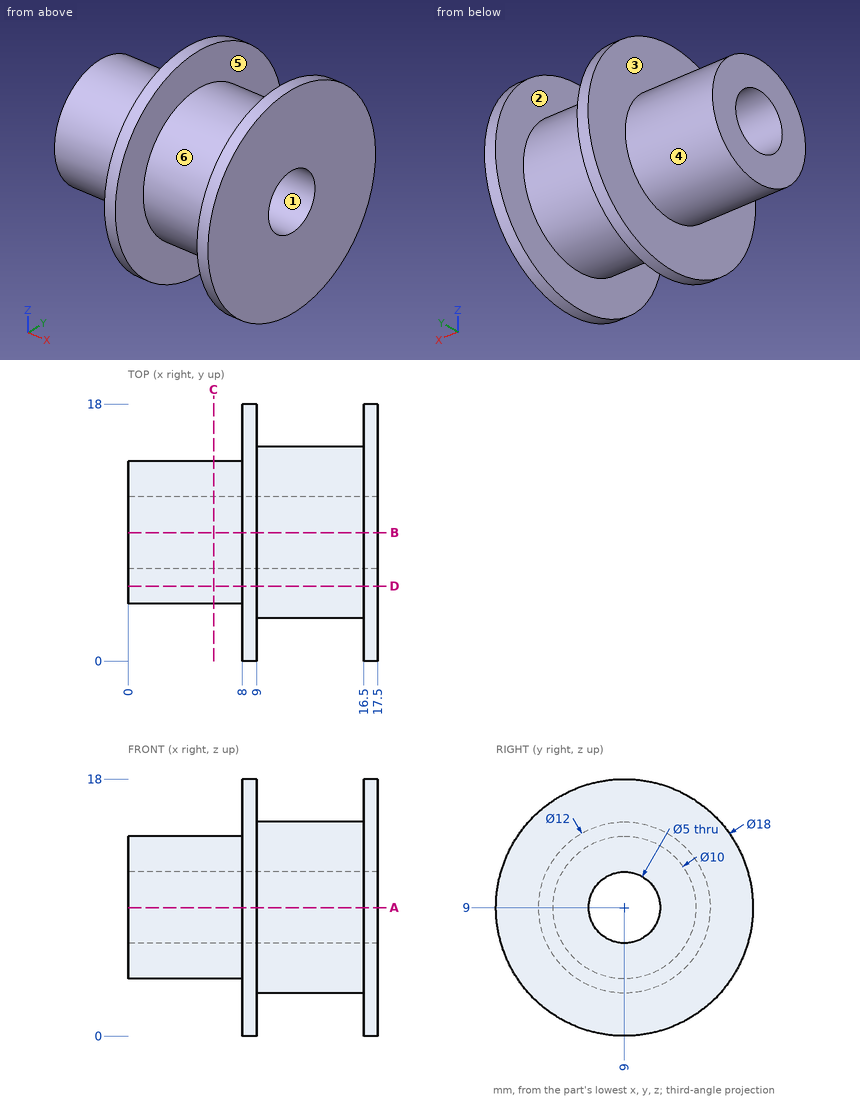
For this review, use the dimensioned drawing (mm, ordinates from the lowest corner) and the shaded views. A direction names the side the tool comes from. Round coordinates to 2 decimals unless told otherwise and drop trailing zeros. Order: outer loops, then holes, each group sorted by start corner. A loop starts at its lowest first (then second) coordinate and runs counter-clockwise, first axis right, second up. Notation, with made-up numbers: (10.25, -23) -> (53.25, -23) arc R15 cw to (53.25, -11) -> close; hole circle Ø3 at (-15.75, 52.5). An arc over 180 degrees is marked (long way). Write item = value, one per line. Start each with the question number.
Item 1: Consider section A-A on z = 9. Write out the cut boundary in (x, y), plus the area to 4 significant figures.
Item 2: Consider section C-C on x = 6. Write out the cut boundary in (y, z), plus the area to 3 significant figures.
Item 3: For the marked faces 1 and 2, list the 3-axis set-ups (+Z, -Z, +X, -X, +Y, -Y) from which the entire face can be reached by the end or side of a thin tool; tool diameter is ignored.
Item 4: Mouldability with a two-part tool opening along X and no side actions: class the marked faces 3, 4, 5 and 6 as released by +X, released by -X, zero draft, split by the parting line, or undercut.
Item 5: Consider section D-D on y = 5.25. Write out the cut boundary in (x, z), plus the area to 3 significant figures.
Item 6: Clearance check with flat-ended pins moving along their axes: pin 1 Ø3 at (x, z) = (5.5, 11.5) entering from +Y; pin 2 Ø5.5 at (y, z) = (7.5, 7.5) entering from -X; pin 3 Ø5 at (x, y) = (3.5, 4.5) entering from -Z; pin 4 Ø4 at (x, y) = (15.5, 2.5) entering from -Z. State where each tip first meets the part, or that it passes through.
Item 7: For line 1 along X through (y, z) = (15, 13.25); line 2 along X through (y, z) = (12.5, 4.5); line 3 along Z through (x, y) = (7.5, 8.25), list the stretches that pass through material, from the lowest coordinate up.
Conclusion:
q1.outline = (0, 4) -> (8, 4) -> (8, 0) -> (9, 0) -> (9, 3) -> (16.5, 3) -> (16.5, 0) -> (17.5, 0) -> (17.5, 6.5) -> (0, 6.5) -> close; (0, 11.5) -> (17.5, 11.5) -> (17.5, 18) -> (16.5, 18) -> (16.5, 15) -> (9, 15) -> (9, 18) -> (8, 18) -> (8, 14) -> (0, 14) -> close
q1.area = 118.5 mm2
q2.outline = circle Ø10 at (9, 9); hole circle Ø5 at (9, 9)
q2.area = 58.9 mm2
q3.face_1 = +X, -X
q3.face_2 = none
q4.face_3 = released by -X
q4.face_4 = zero draft
q4.face_5 = undercut
q4.face_6 = undercut
q5.outline = (0, 5.69) -> (8, 5.69) -> (8, 0.82) -> (9, 0.82) -> (9, 4.32) -> (16.5, 4.32) -> (16.5, 0.82) -> (17.5, 0.82) -> (17.5, 17.18) -> (16.5, 17.18) -> (16.5, 13.68) -> (9, 13.68) -> (9, 17.18) -> (8, 17.18) -> (8, 12.31) -> (0, 12.31) -> close
q5.area = 156 mm2
q6.pin_1 = 13.9
q6.pin_2 = 0
q6.pin_3 = 4.42
q6.pin_4 = 1.37
q7.line_1 = 8 to 9, 16.5 to 17.5
q7.line_2 = 8 to 17.5
q7.line_3 = 4.06 to 6.62, 11.38 to 13.94
